Autodesk Inventor part; units mm, degrees
ref_plane "YZ Plane" through (0, 0, 0) normal (1, 0, 0) x (0, 1, 0)
ref_plane "XZ Plane" through (0, 0, 0) normal (0, 1, 0) x (-1, 0, 0)
ref_plane "XY Plane" through (0, 0, 0) normal (0, 0, 1) x (1, 0, 0)
sketch "Sketch1" plane through (0, 0, 0) normal (0, 0, 1) x (1, 0, 0)
  line L0 (0, 0) -> (0, 4438.8737)
  line L1 (0, 4438.8737) -> (100, 4438.8737)
  line L2 (100, 4438.8737) -> (200, 0)
  line L3 (200, 0) -> (0, 0)
  circle A0 centre (0, 0) radius 30
  line L4 (0, 1479.6246) -> (166.6667, 1479.6246)
  line L5 (0, 2959.2492) -> (133.3333, 2959.2492)
  circle A1 centre (0, 1479.6246) radius 30
  circle A2 centre (0, 2959.2492) radius 30
  line L6 (190.8761, 405) -> (120.8761, 405)
  line L7 (120.8761, 405) -> (120.8761, 410)
  line L8 (120.8761, 410) -> (190.8761, 410)
  line L9 (190.8761, 410) -> (190.8761, 405)
  line L10 (109.6148, 909.8732) -> (179.6148, 909.8732)
  line L11 (179.6148, 904.8732) -> (109.6148, 904.8732)
  line L12 (109.6148, 904.8732) -> (109.6148, 909.8732)
  line L13 (179.6148, 909.8732) -> (179.6148, 904.8732)
  line L14 (98.3535, 1409.7463) -> (168.3535, 1409.7463)
  line L15 (168.3535, 1404.7463) -> (98.3535, 1404.7463)
  line L16 (98.3535, 1404.7463) -> (98.3535, 1409.7463)
  line L17 (168.3535, 1409.7463) -> (168.3535, 1404.7463)
  line L18 (87.0923, 1909.6195) -> (157.0923, 1909.6195)
  line L19 (157.0923, 1904.6195) -> (87.0923, 1904.6195)
  line L20 (87.0923, 1904.6195) -> (87.0923, 1909.6195)
  line L21 (157.0923, 1909.6195) -> (157.0923, 1904.6195)
  line L22 (75.831, 2409.4927) -> (145.831, 2409.4927)
  line L23 (145.831, 2404.4927) -> (75.831, 2404.4927)
  line L24 (75.831, 2404.4927) -> (75.831, 2409.4927)
  line L25 (145.831, 2409.4927) -> (145.831, 2404.4927)
  line L26 (64.5698, 2909.3658) -> (134.5698, 2909.3658)
  line L27 (134.5698, 2904.3658) -> (64.5698, 2904.3658)
  line L28 (64.5698, 2904.3658) -> (64.5698, 2909.3658)
  line L29 (134.5698, 2909.3658) -> (134.5698, 2904.3658)
  line L30 (53.3085, 3409.239) -> (123.3085, 3409.239)
  line L31 (123.3085, 3404.239) -> (53.3085, 3404.239)
  line L32 (53.3085, 3404.239) -> (53.3085, 3409.239)
  line L33 (123.3085, 3409.239) -> (123.3085, 3404.239)
  line L34 (42.0472, 3909.1122) -> (112.0472, 3909.1122)
  line L35 (112.0472, 3904.1122) -> (42.0472, 3904.1122)
  line L36 (42.0472, 3904.1122) -> (42.0472, 3909.1122)
  line L37 (112.0472, 3909.1122) -> (112.0472, 3904.1122)
  line L38 (0, 1629.6246) -> (163.2874, 1629.6246)
  line L39 (0, 3079.2492) -> (130.6299, 3079.2492)
  point P0 (30, 2959.2492)
  point P1 (0, 2929.2492)
  point P2 (0, 1509.6246)
  point P3 (0, 1449.6246)
  point P4 (0, 30)
  point P5 (30, 0)
  point P6 (190.7634, 410)
  point P7 (179.5022, 909.8732)
  point P8 (168.3535, 1404.7463)
  point P9 (168.2409, 1409.7463)
  point P10 (30, 1479.6246)
  point P11 (157.0923, 1904.6195)
  point P12 (156.9796, 1909.6195)
  point P13 (145.831, 2404.4927)
  point P14 (145.7184, 2409.4927)
  point P15 (134.5698, 2904.3658)
  point P16 (134.4571, 2909.3658)
  point P17 (0, 2989.2492)
  dimension "d65" = 100
  dimension "d67" = 200
  dimension "d68" = 60
  dimension "d69" = 1480
  dimension "d70" = 1480
  dimension "d71" = 1480
  dimension "d72" = 5
  dimension "d73" = 70
  dimension "d74" = 410
  dimension "d77" = 500
  dimension "d82" = 120
  dimension "d83" = 150
extrude "Plate3" add sketch "Sketch1" along normal blind 4 contours L39 L2 L5 A2 L0 | L5 L2 L26 L28 L27 L22 L24 L23 L18 L20 L19 L38 L0 A2 | L38 L2 L4 A1 L0
chamfer "Corner Chamfer2" distance 3 angle 45 6 edges at (157.0923, 1904.6195, 2) (156.9796, 1909.6195, 2) (145.831, 2404.4927, 2) (145.7184, 2409.4927, 2) (134.5698, 2904.3658, 2) (134.4571, 2909.3658, 2)
equation "\"BendRadius\" = Thickness"
equation "\"BendReliefWidth\" = Thickness"
equation "\"BendReliefDepth\" = 0.5 * Thickness"
equation "\"CornerReliefSize\" = 4 * Thickness"
equation "\"MinimumRemnant\" = 2 * Thickness"
equation "\"TransitionRadius\" = BendRadius"
equation "\"JacobiRadiusSize\" = BendRadius"
equation "\"GapSize\" = Thickness"
properties part number "GBK 3212 central second rib_CPY" material "Steel"
Design review of the part built by this model. Coordinates are the model's own, in mm. Give positions to 0.01 mm unless a question says otherwise; leave off trailing zeros. Write each loop counter-clockwise with the first axis right and the second up, starting at its lowest first coordinate (ties: lowest second). Pieces come first, ordered by that corner, then holes. Notation, with made-up numbers: (23, 11) - (64, 11) arc R13 ccw to (64, 26) - close; hole circle Ø9 at (77.25, -25.75). An arc over 180 degrees is marked (long way). Return JSON: item names as keys, results as strings. Group by question number.
(1) We need section B-B, the plane y = 2573. Give the boundary of the cut face in (x, z).
(2) We need section C-C, the plane y = 2304. Give the boundary of the cut face in (x, z), then the cut area to 3 significant figures.
(3) To check wall thickness, follow probe 1 along Y at (x, z) = (98.5, 2.2); probe 2 along Y at (x, z) = (76.5, 1.95); probe 3 along Y at (x, z) = (66.5, 0.5). State the ranges of each line that lie inside material, in increasing order.
(4) Insertion check: pin 1 (2 mm diameter, centred on y = 2406, z = 1.5, fed in from +X); pin 2 (2 mm diameter, centred on y = 2458.5, z = 0.5, fed in from +X). Each pin has a flat end and moves straight along its axis. Give the tip position at first contact, or say it passes through.
(5) Mouldability with a two-part tool opening along Y and no side actions: class faces 1 (the cylindrical face through (29.993, 2959.909, 1.972)), 2 (the flat face through (82, 2291, 4)), 3 (the cylindrical face through (20.98, 1501.07, 1.97)) as +Y half, -Y half, draft (parallel to the pull), parting line (faces both ways), or undercut.
(6) We need section A-A, the plane z = 2.05. Give the boundary of the cut face in (x, y), then the cut area to 3 significant figures.
Reported:
{
 "1": {"outline": "(0, 0) - (142.03, 0) - (142.03, 4) - (0, 4) - close"},
 "2": {"outline": "(0, 0) - (148.09, 0) - (148.09, 4) - (0, 4) - close", "area": "592 mm2"},
 "3": {"probe 1": "y = 1479.62 to 1904.62, 1909.62 to 2404.49, 2409.49 to 2904.37, 2909.37 to 3079.25", "probe 2": "y = 1479.62 to 2404.49, 2409.49 to 2904.37, 2909.37 to 3079.25", "probe 3": "y = 1479.62 to 2904.37, 2909.37 to 3079.25"},
 "4": {"pin 1": "stops at x = 75.83", "pin 2": "stops at x = 144.64"},
 "5": {"face 1": "undercut", "face 2": "draft", "face 3": "-Y half"},
 "6": {"outline": "(0, 1509.62) arc R30 cw to (30, 1479.62) - (166.67, 1479.62) - (157.16, 1901.62) - (154.09, 1904.62) - (87.09, 1904.62) - (87.09, 1909.62) - (153.98, 1909.62) - (156.91, 1912.62) - (145.9, 2401.49) - (142.83, 2404.49) - (75.83, 2404.49) - (75.83, 2409.49) - (142.72, 2409.49) - (145.65, 2412.49) - (134.64, 2901.37) - (131.57, 2904.37) - (64.57, 2904.37) - (64.57, 2909.37) - (131.46, 2909.37) - (134.39, 2912.37) - (130.63, 3079.25) - (0, 3079.25) - (0, 2989.25) arc R30 cw to (0, 2929.25) - close", "area": "235,000 mm2"}
}
